```python
from build123d import *

# Parameters (mm, degrees)
F1_DEPTH = 7.5
F2_W     = 8
F2_H     = 1.25
F3_DEPTH = 25
F4_W     = 0.5
F4_H     = 0.5
F5_DEPTH = 25
F6_W     = 6
F6_H     = 1
F7_DEPTH = 1


with BuildPart() as f1:
    # F0 (on Top) → F1 (new body)
    with BuildSketch(Plane.XY):
        Polygon((0, 3.5), (0, 0), (6, 0), (6, 11.5), (5, 11.5), (5, 3.5), align=None)
    extrude(amount=F1_DEPTH)

    # F2 (on face) → F3 (cut)
    with BuildSketch(Plane(origin=(5, 0, 0), x_dir=(0, -1, 0), z_dir=(-1, 0, 0))):
        with Locations((-7.5, 0.625)):
            Rectangle(F2_W, F2_H)
        with Locations((-7.5, 6.875)):
            Rectangle(F2_W, F2_H)
    extrude(amount=-F3_DEPTH, mode=Mode.SUBTRACT)

    # F4 (on face) → F5 (cut)
    with BuildSketch(Plane(origin=(0, 3.5, 0), x_dir=(-1, 0, 0), z_dir=(0, 1, 0))):
        with Locations((-3.75, 6)):
            Rectangle(F4_W, F4_H)
        with Locations((-3.75, 1.5)):
            Rectangle(F4_W, F4_H)
        with Locations((-3.75, 3.75)):
            Rectangle(F4_W, F4_H)
    extrude(amount=-F5_DEPTH, mode=Mode.SUBTRACT)

    # F6 (on face) → F7 (cut)
    with BuildSketch(Plane.XZ):
        with Locations((3, 6)):
            Rectangle(F6_W, F6_H)
        with Locations((3, 3.75)):
            Rectangle(F6_W, F6_H)
        with Locations((3, 1.5)):
            Rectangle(F6_W, F6_H)
    extrude(amount=-F7_DEPTH, mode=Mode.SUBTRACT)


solid = f1.part
```
Check sheet for the modelled part. Datum: model origin and axes. Units: mm. A direction names the side the tool comes from. Coordinates: 2 decimals unless noted, no trailing zeros. Write each loop counter-clockwise with the first axis right and the second up, starting at its lowest first coordinate (ties: lowest second). Pieces come first, ordered by that corner, then holes. Notation, with made-up numbers: M 44.25,72.5 L 76.25,72.5 A12 ccw 76.25,91.5 Z; hole C 19.25,64 d1. An arc over 180 degrees is marked long. Write item = value, one per line. Start each with the question number.
1. Thickness scan on probe 1 along Y at (x, z) = (2.35, 3.5); probe 2 along Y at (x, z) = (5.35, 1.5); probe 3 along X at (y, z) = (5, 5.75). Record the ranges inside material, lowest first.
2. Sectioned sample at C-C (z = 2.25). Record the cut outline in (x, y), then the cut area to 3 significant figures.
3. Sectioned sample at D-D (y = 9.25). Record the cut outline in (x, z), then the cut area to 3 significant figures.
4. Sectioned sample at A-A (y = 1.25). Record the cut outline in (x, z), then the cut area to 4 significant figures.
5. Tool access check on faces 1 (the flat face through (0, 2, 4)), 2 (the flat face through (5, 8, 4)), 3 (the flat face through (3, 1, 4)). Record the directions out of +Z, -Z, +X, -X, +Y, -Y that give a thin tool (end or side, any length) a straight path to the whole face; none if there is none.
6. Mould release check, pull along Z, two halves, no side actions. Record for faces 4 (the flat face through (5.5, 7.6, 1.25)), 5 (the flat face through (3, 2, 7.5)), 6 (the flat face through (3, 0.5, 2)), 7 (the flat face through (3, 0, 7)): pulls with the +Z half, pulls with the -Z half, needs draft (parallel to the pull), parting line crosses it, or undercut.
7. Go/stop test with flat-tipped pins: pin 1 (0.8 mm diameter, centred on x = 5.5, y = 7.5, fed in from -Z); pin 2 (1 mm diameter, centred on x = 3, z = 1, fed in from +Y). Record where each tip stops, or that it passes through.
8. Sectioned sample at B-B (x = 0.45). Record the cut outline in (y, z), then the cut area to 4 significant figures.
The answers:
q1.probe_1 = 1 to 3.5
q1.probe_2 = 1 to 11.5
q1.probe_3 = 5 to 6
q2.outline = M 0,0 L 6,0 L 6,11.5 L 5,11.5 L 5,3.5 L 0,3.5 Z
q2.area = 29.0 mm²
q3.outline = M 5,1.25 L 6,1.25 L 6,6.25 L 5,6.25 Z
q3.area = 5.00 mm²
q4.outline = M 0,0 L 6,0 L 6,7.5 L 0,7.5 Z; hole M 3.5,1.25 L 4,1.25 L 4,1.75 L 3.5,1.75 Z; hole M 3.5,3.5 L 4,3.5 L 4,4 L 3.5,4 Z; hole M 3.5,5.75 L 4,5.75 L 4,6.25 L 3.5,6.25 Z
q4.area = 44.25 mm²
q5.face_1 = +Z, -Z, -X, +Y, -Y
q5.face_2 = +Z, -Z, -X, +Y
q5.face_3 = +X, -X, -Y
q6.face_4 = pulls with the -Z half
q6.face_5 = pulls with the +Z half
q6.face_6 = undercut
q6.face_7 = needs draft
q7.pin_1 = 1.25
q7.pin_2 = 3.5
q8.outline = M 0,0 L 3.5,0 L 3.5,7.5 L 0,7.5 L 0,6.5 L 1,6.5 L 1,5.5 L 0,5.5 L 0,4.25 L 1,4.25 L 1,3.25 L 0,3.25 L 0,2 L 1,2 L 1,1 L 0,1 Z
q8.area = 23.25 mm²
